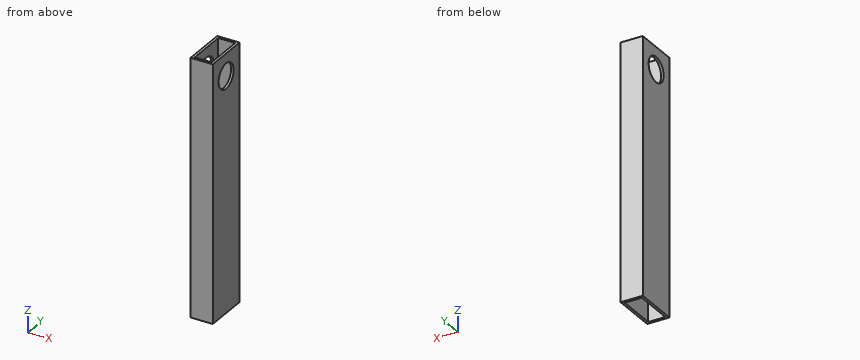
```python
from build123d import *

# Parameters (mm, degrees)
F_2X1_BLANK_EXTRUSION_OUTLINE_W   = 25.4
F_2X1_BLANK_EXTRUSION_OUTLINE_H   = 50.8
F_2X1_BLANK_EXTRUSION_OUTLINE_W_2 = 19.558
F_2X1_BLANK_EXTRUSION_OUTLINE_H_2 = 44.958
F_2X1_BLANK_EXTRUSION_DEPTH       = 292.1
CUT_EXTRUDE1_DEPTH                = 295.300407747
CUT_EXTRUDE1_DEPTH_BACK           = 295.300407747
SKETCH1_R                         = 14.2875


# Read off the part's stored shape, not the designer's step: 2x1 blank extrusion
with BuildPart() as part:
    # 2x1 blank extrusion outline → 2x1 blank extrusion (new body)
    with BuildSketch(Plane.XY):
        Rectangle(F_2X1_BLANK_EXTRUSION_OUTLINE_W, F_2X1_BLANK_EXTRUSION_OUTLINE_H)
        Rectangle(F_2X1_BLANK_EXTRUSION_OUTLINE_W_2, F_2X1_BLANK_EXTRUSION_OUTLINE_H_2, mode=Mode.SUBTRACT)
    extrude(amount=F_2X1_BLANK_EXTRUSION_DEPTH)

    # Sketch1 → Cut-Extrude1 (cut, two sides: drawn at the far end of the back side and taken through both)
    with BuildSketch(Plane(origin=(12.7, 0, 0), x_dir=(0, 0, -1), z_dir=(1, 0, 0)).offset(-CUT_EXTRUDE1_DEPTH_BACK)):
        with Locations(Location((-266.7, 0, 0), (0, 0, 180))):
            Circle(SKETCH1_R)
    extrude(amount=CUT_EXTRUDE1_DEPTH + CUT_EXTRUDE1_DEPTH_BACK, mode=Mode.SUBTRACT)


solid = part.part
```
Design review of the part built by this model. Coordinates are the model's own, in mm. Give positions to 0.01 mm unless a question says otherwise; leave off trailing zeros. Order: outer loops, then holes, each group sorted by start corner. A loop starts at its lowest first (then second) coordinate and runs counter-clockwise, first axis right, second up. Notation, with made-up numbers: (48.5, 21.25) -> (57.5, 21.25) arc R16 cw to (57.5, 47.25) -> close; hole circle Ø5 at (14, 25.25). An arc over 180 degrees is marked (long way). Write item = value, one per line. Start each with the question number.
(1) We need section D-D on z = 266.7. Write out the cut boundary in (x, y), plus the area to 3 significant figures.
(2) We need section A-A on x = -7. Write out the cut boundary in (y, z).
(3) For pin 1 (6 mm diameter, centred on x = -5.5, y = 10.5, fed in from -Z), flat-tipped, find the tip position at first contact; note if it passes through.
(4) We need section C-C on z = 60.5. Write out the cut boundary in (x, y), plus the area to 3 significant figures.
(5) We need section B-B on y = 0. Write out the cut boundary in (x, z).
(6) To check wall thickness, follow line 1 along Y through (x, z) = (0.5, 229); line 2 along X through (y, z) = (1.5, 83); line 3 along Y through (x, z) = (11.4, 266.7). State the ranges of each line that lie inside material, in increasing order.
Numbers:
q1.outline = (-12.7, -25.4) -> (12.7, -25.4) -> (12.7, -14.29) -> (9.78, -14.29) -> (9.78, -22.48) -> (-9.78, -22.48) -> (-9.78, -14.29) -> (-12.7, -14.29) -> close; (-12.7, 14.29) -> (-9.78, 14.29) -> (-9.78, 22.48) -> (9.78, 22.48) -> (9.78, 14.29) -> (12.7, 14.29) -> (12.7, 25.4) -> (-12.7, 25.4) -> close
q1.area = 244 mm^2
q2.outline = (-25.4, 0) -> (-22.48, 0) -> (-22.48, 292.1) -> (-25.4, 292.1) -> close; (22.48, 0) -> (25.4, 0) -> (25.4, 292.1) -> (22.48, 292.1) -> close
q3.pin_1 = through
q4.outline = (-12.7, -25.4) -> (12.7, -25.4) -> (12.7, 25.4) -> (-12.7, 25.4) -> close; hole (-9.78, -22.48) -> (9.78, -22.48) -> (9.78, 22.48) -> (-9.78, 22.48) -> close
q4.area = 411 mm^2
q5.outline = (-12.7, 0) -> (-9.78, 0) -> (-9.78, 252.41) -> (-12.7, 252.41) -> close; (-12.7, 280.99) -> (-9.78, 280.99) -> (-9.78, 292.1) -> (-12.7, 292.1) -> close; (9.78, 0) -> (12.7, 0) -> (12.7, 252.41) -> (9.78, 252.41) -> close; (9.78, 280.99) -> (12.7, 280.99) -> (12.7, 292.1) -> (9.78, 292.1) -> close
q6.line_1 = -25.4 to -22.48, 22.48 to 25.4
q6.line_2 = -12.7 to -9.78, 9.78 to 12.7
q6.line_3 = -25.4 to -14.29, 14.29 to 25.4
